Input: dimensioned drawing with shaded views. Units: mm. Origin: part minimum x, y, z. Give positions to 0.01 mm unless a question says otherwise; leave off trailing zeros. Write each loop counter-clockwise with the first axis right and the second up, starting at its lowest first coordinate (ties: lowest second). Pieces come first, ordered by that corner, then holes. Notation, with made-up numbers: M 56,-23.5 L 61,-23.5 A19 cw 61,13.5 Z; hole C 84.25,30 d6. An arc over 180 degrees is marked long. Answer as a JSON object with one key per item and string values.
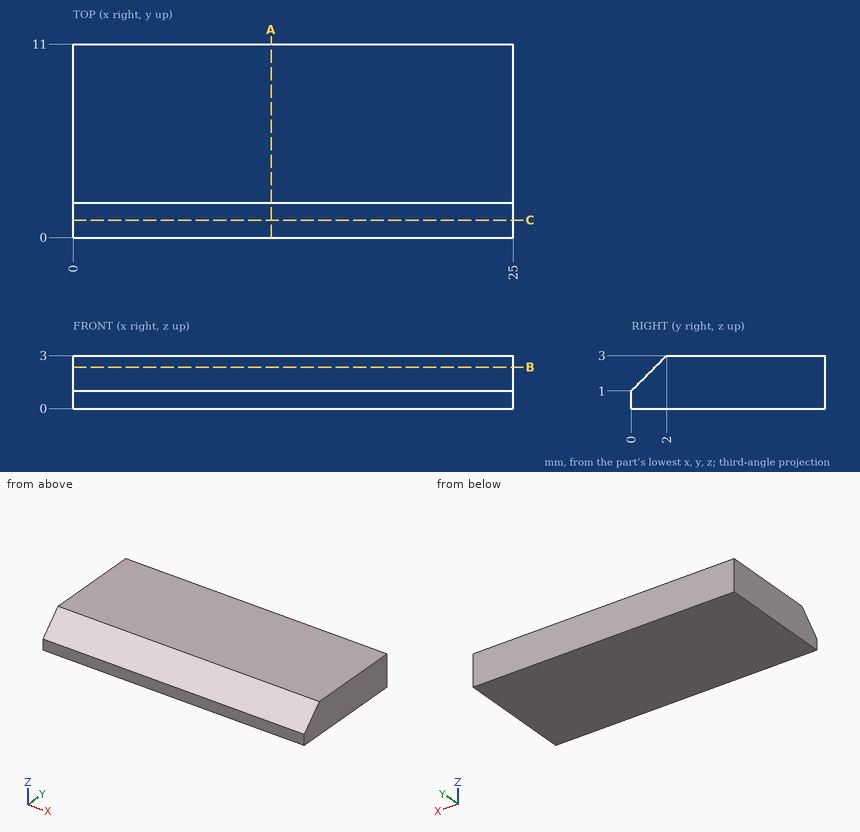
1) Line query: line 1 (Y direction, x = 4, z = 1.4); line 2 (Z direction, x = 7.75, y = 1.25); line 3 (Y direction, x = 23, z = 2.1). Output: solid intervals per line, ascending. Write a range as from..to.
Geometry check:
{"line 1": "y = 0.4..11", "line 2": "z = 0..2.25", "line 3": "y = 1.1..11"}
2) Cut plane B-B on z = 2.35. Return loops of the section in (x, y).
Geometry check:
{"outline": "M 0,1.35 L 25,1.35 L 25,11 L 0,11 Z"}
3) Cut plane A-A on x = 11.25. Return loops of the section in (y, z).
Geometry check:
{"outline": "M 0,0 L 11,0 L 11,3 L 2,3 L 0,1 Z"}
4) Cut plane C-C on y = 1. Return loops of the section in (x, z).
Geometry check:
{"outline": "M 0,0 L 25,0 L 25,2 L 0,2 Z"}
